Geometry check sheet. Reference: the model listing, model coordinates, mm. Round coordinates to 2 decimals unless told otherwise and drop trailing zeros. Write each loop counter-clockwise with the first axis right and the second up, starting at its lowest first coordinate (ties: lowest second). Pieces come first, ordered by that corner, then holes.
from build123d import *

# Parameters (mm, degrees)
SALIENTE_EXTRUIR1_DEPTH = 3
REDONDEO1_R             = 10
CROQUIS2_R              = 1.5
CROQUIS2_R_2            = 2
CROQUIS2_R_3            = 2.05
CROQUIS2_W              = 42
CROQUIS2_H              = 20
CORTAR_EXTRUIR1_DEPTH   = 135.610141171
CROQUIS3_W              = 4
CROQUIS3_H              = 14.636342218
CORTAR_EXTRUIR2_DEPTH   = 135.610141171
CROQUIS4_W              = 44
CROQUIS4_H              = 22
CORTAR_EXTRUIR3_DEPTH   = 131.820067673
CORTAR_EXTRUIR4_DEPTH   = 131.820067673
REDONDEO2_R             = 20
CORTAR_EXTRUIR5_DEPTH   = 10
REDONDEO3_R             = 10
CROQUIS7_W              = 14.636342218
CROQUIS7_H              = 3
SALIENTE_EXTRUIR2_DEPTH = 2
CROQUIS8_W              = 14.636342218
CROQUIS8_H              = 3
SALIENTE_EXTRUIR3_DEPTH = 2
CROQUIS10_R             = 2
CORTAR_EXTRUIR7_DEPTH   = 133.713564137


with BuildPart() as part:
    # Croquis1 → Saliente-Extruir1 (new body)
    with BuildSketch(Plane(origin=(0, 0, 0), x_dir=(1, 0, 0), z_dir=(0, 1, 0))):
        Polygon((-88.1, 42.318171109), (88.1, 42.318171109), (108.1, 22.318171109), (127.75, 22.318171109), (127.75, 7.681828891), (105.75, 7.681828891), (77.75, -42.318171109), (-77.75, -42.318171109), (-105.75, 7.681828891), (-127.75, 7.681828891), (-127.75, 22.318171109), (-108.1, 22.318171109), align=None)
    extrude(amount=SALIENTE_EXTRUIR1_DEPTH)

    # Redondeo1
    redondeo1_edges = [part.edges().sort_by_distance(p)[0] for p in [
        (-88.1, 1.5, -42.318171109),
        (88.1, 1.5, -42.318171109),
        (108.1, 1.5, -22.318171109),
        (105.75, 1.5, -7.681828891),
        (77.75, 1.5, 42.318171109),
        (-77.75, 1.5, 42.318171109),
        (-105.75, 1.5, -7.681828891),
        (-108.1, 1.5, -22.318171109),
    ]]
    fillet(redondeo1_edges, radius=REDONDEO1_R)

    # Croquis2 → Cortar-Extruir1 (cut, through all)
    with BuildSketch(Plane(origin=(0, 3, 0), x_dir=(1, 0, 0), z_dir=(0, 1, 0))):
        with Locations(Location((70, -27.318171109, 0), (0, 0, 270))):
            Circle(CROQUIS2_R)
        with Locations(Location((-70, -27.318171109, 0), (0, 0, 270))):
            Circle(CROQUIS2_R)
        with Locations(Location((-119.996067812, 15, 0), (0, 0, 270))):
            Circle(CROQUIS2_R)
        with Locations(Location((119.996067812, 15, 0), (0, 0, 270))):
            Circle(CROQUIS2_R)
        with Locations(Location((-11.5, -14.318171109, 0), (0, 0, 270))):
            Circle(CROQUIS2_R_2)
        with Locations(Location((11.5, -14.318171109, 0), (0, 0, 270))):
            Circle(CROQUIS2_R_2)
        with Locations(Location((-11.5, -37.318171109, 0), (0, 0, 270))):
            Circle(CROQUIS2_R_2)
        with Locations(Location((11.5, -37.318171109, 0), (0, 0, 270))):
            Circle(CROQUIS2_R_2)
        with Locations(Location((-61, 7.318171109, 0), (0, 0, 270))):
            Circle(CROQUIS2_R_3)
        with Locations(Location((-11, 7.318171109, 0), (0, 0, 270))):
            Circle(CROQUIS2_R_3)
        with Locations(Location((-61, 13.318171109, 0), (0, 0, 270))):
            Circle(CROQUIS2_R_3)
        with Locations(Location((-61, 1.318171109, 0), (0, 0, 270))):
            Circle(CROQUIS2_R_3)
        with Locations(Location((-11, 13.318171109, 0), (0, 0, 270))):
            Circle(CROQUIS2_R_3)
        with Locations(Location((-11, 1.318171109, 0), (0, 0, 270))):
            Circle(CROQUIS2_R_3)
        with Locations((-36, 7.318171109)):
            Rectangle(CROQUIS2_W, CROQUIS2_H)
    extrude(amount=-CORTAR_EXTRUIR1_DEPTH, mode=Mode.SUBTRACT)

    # Croquis3 → Cortar-Extruir2 (cut, through all)
    with BuildSketch(Plane(origin=(0, 3, 0), x_dir=(1, 0, 0), z_dir=(0, 1, 0))):
        with Locations((-125.75, 15)):
            Rectangle(CROQUIS3_W, CROQUIS3_H)
        with Locations((125.75, 15)):
            Rectangle(CROQUIS3_W, CROQUIS3_H)
    extrude(amount=-CORTAR_EXTRUIR2_DEPTH, mode=Mode.SUBTRACT)

    # Croquis4 → Cortar-Extruir3 (cut, through all)
    with BuildSketch(Plane(origin=(0, 3, 0), x_dir=(1, 0, 0), z_dir=(0, 1, 0))):
        with Locations((-36, 7.318171109)):
            Rectangle(CROQUIS4_W, CROQUIS4_H)
    extrude(amount=-CORTAR_EXTRUIR3_DEPTH, mode=Mode.SUBTRACT)

    # Croquis5 → Cortar-Extruir4 (cut, through all)
    with BuildSketch(Plane(origin=(0, 3, 0), x_dir=(1, 0, 0), z_dir=(0, 1, 0))):
        Polygon((-63.75, 42.318171109), (-38.75, 32.318171109), (38.75, 32.318171109), (63.75, 42.318171109), align=None)
    extrude(amount=-CORTAR_EXTRUIR4_DEPTH, mode=Mode.SUBTRACT)

    # Redondeo2
    redondeo2_edges = [part.edges().sort_by_distance(p)[0] for p in [
        (-63.75, 1.5, -42.318171109),
        (63.75, 1.5, -42.318171109),
        (38.75, 1.5, -32.318171109),
        (-38.75, 1.5, -32.318171109),
    ]]
    fillet(redondeo2_edges, radius=REDONDEO2_R)

    # Croquis6 → Cortar-Extruir5 (cut)
    with BuildSketch(Plane(origin=(0, 3, 0), x_dir=(1, 0, 0), z_dir=(0, 1, 0))):
        Polygon((-34.898351929, 32.318171109), (-98.1, 32.318171109), (-98.1, 50.604425951), (105.42793471, 50.604425951), (105.42793471, 32.318171109), align=None)
    extrude(amount=-CORTAR_EXTRUIR5_DEPTH, mode=Mode.SUBTRACT)

    # Redondeo3
    redondeo3_edges = [part.edges().sort_by_distance(p)[0] for p in [
        (98.1, 1.5, -32.318171109),
        (-98.1, 1.5, -32.318171109),
    ]]
    fillet(redondeo3_edges, radius=REDONDEO3_R)

    # Croquis7 → Saliente-Extruir2 (add)
    with BuildSketch(Plane.ZY.offset(123.75)):
        with Locations((-15, 1.5)):
            Rectangle(CROQUIS7_W, CROQUIS7_H)
    extrude(amount=SALIENTE_EXTRUIR2_DEPTH)

    # Croquis8 → Saliente-Extruir3 (add)
    with BuildSketch(Plane(origin=(123.75, 0, 0), x_dir=(0, 0, -1), z_dir=(1, 0, 0))):
        with Locations((15, 1.5)):
            Rectangle(CROQUIS8_W, CROQUIS8_H)
    extrude(amount=SALIENTE_EXTRUIR3_DEPTH)

    # Croquis10 → Cortar-Extruir7 (cut, through all)
    with BuildSketch(Plane(origin=(0, 3, 0), x_dir=(1, 0, 0), z_dir=(0, 1, 0))):
        with Locations(Location((-80, 26.318171109, 0), (0, 0, 270))):
            Circle(CROQUIS10_R)
        with Locations(Location((80, 26.318171109, 0), (0, 0, 270))):
            Circle(CROQUIS10_R)
    extrude(amount=-CORTAR_EXTRUIR7_DEPTH, mode=Mode.SUBTRACT)


solid = part.part
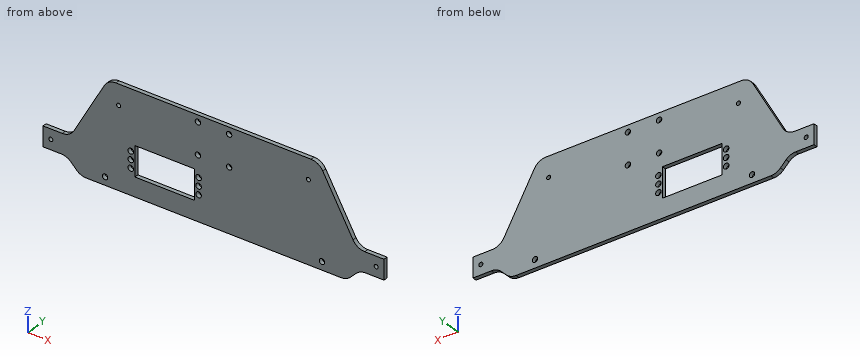
1. Depth check by flat-ended pin: pin 1 Ø0.9 at (x, y) = (-119.5, 1) entering from +Z; pin 2 Ø1.5 at (x, y) = (118.5, 2) entering from -Z. Enter the tip coordinate at first touch or a pass-through.
2. Section check D-D (x = 97.5). Record the cut outline in (y, z), plus the area to 3 significant figures.
3. Section check C-C (y = 1.7). State how many separate pieces and enclosed holes the cut face has, plus the area to 3 significant figures.
4. Scan lines: line 1 along Z through (x, y) = (-40.5, 2.55); line 2 along X through (y, z) = (1.6, 27.5); line 3 along X through (y, z) = (0.65, -15). Record each from-to range of solid material in increasing order.
5. Section check B-B (z = 7). Record the cut outline in (x, y), plus the area to 3 significant figures.
6. Section check A-A (x = -48.5). Record the cut outline in (y, z).
Results below:
1. pin 1: stops at z = -7.68
1. pin 2: stops at z = -22.32
2. outline: (0, -31.67) - (3, -31.67) - (3, 7.05) - (0, 7.05) - close
2. area: 116 mm2
3. separate pieces: 1
3. enclosed holes: 17
3. area: 13,800 mm2
4. line 1: z = -32.32 to -18.32, 3.68 to 42.32
4. line 2: x = -86.05 to -71.49, -68.51 to 68.51, 71.49 to 86.05
4. line 3: x = -125.75 to -121.5, -118.5 to -62.17, -59.83 to -58, -14 to -12.17, -9.83 to 118.5, 121.5 to 125.75
5. outline: (-97.53, 0) - (97.53, 0) - (97.53, 3) - (-97.53, 3) - close
5. area: 585 mm2
6. outline: (0, -32.32) - (3, -32.32) - (3, -18.32) - (0, -18.32) - close; (0, 3.68) - (3, 3.68) - (3, 42.32) - (0, 42.32) - close
